from build123d import *

# Parameters (mm, degrees)
FILLET1_R = 1.5


with BuildPart() as part:
    # Sketch1 → Revolve1 (revolve)
    with BuildSketch(Plane.XY):
        with BuildLine():
            Line((29.062623268, -28.998781924), (35, -87.278860618))
            Line((35, -87.278860618), (50, -87.278860618))
            Line((50, -87.278860618), (50, -90.278860618))
            Line((50, -90.278860618), (70, -90.278860618))
            Line((70, -90.278860618), (70, -70.278860618))
            Line((70, -70.278860618), (50, -70.278860618))
            ThreePointArc((50, -70.278860618), (44.343145751, -67.935714867), (42, -62.278860618))
            Line((42, -62.278860618), (32, 52.5))
            Line((32, 52.5), (35, 52.5))
            Line((35, 52.5), (35, 92.5))
            Line((35, 92.5), (25, 92.5))
            Line((25, 92.5), (25, 17.342006044))
            Line((25, 17.342006044), (29.062623268, -28.998781924))
        make_face()
    revolve(axis=Axis((0, -90.278860618, 0), (0, 1, 0)))

    # Fillet1
    fillet1_edges = [part.edges().sort_by_distance(p)[0] for p in [
        (-50, -87.278860618, 0),
    ]]
    fillet(fillet1_edges, radius=FILLET1_R)


solid = part.part
Can you work these out from the model? Positions are in its coordinate system, mm. A direction names the side the tool comes from. Give positions to 0.01 mm unless a question says otherwise; leave off trailing zeros. Loops run counter-clockwise (first coordinate to the right, second up) from the corner with the lowest first, then second, coordinate; pieces in that order, holes last. Notation, with made-up numbers: (16, 7) -> (41, 7) arc R16 ccw to (41, 31) -> close; hole circle Ø1 at (35.25, 36). An arc over 180 degrees is marked (long way). Write item = value, one per line.
1) Suppose I cut it at A-A on z = 0. Write out the boundary of the cut face in (x, y).
Check result:
outline = (-70, -90.28) -> (-50, -90.28) -> (-50, -88.78) arc R1.5 cw to (-48.5, -87.28) -> (-35, -87.28) -> (-29.06, -29) -> (-25, 17.34) -> (-25, 92.5) -> (-35, 92.5) -> (-35, 52.5) -> (-32, 52.5) -> (-42, -62.28) arc R8 cw to (-50, -70.28) -> (-70, -70.28) -> close; (25, 17.34) -> (29.06, -29) -> (35, -87.28) -> (48.5, -87.28) arc R1.5 cw to (50, -88.78) -> (50, -90.28) -> (70, -90.28) -> (70, -70.28) -> (50, -70.28) arc R8 cw to (42, -62.28) -> (32, 52.5) -> (35, 52.5) -> (35, 92.5) -> (25, 92.5) -> close
2) Thinking about a two-plate mould opening in X: for faces 1 (the flat face through (-48, -70.279, -17)), 2 (the conical face through (19.85, -4.09, -31.14)), 3 (the cylindrical face through (47.69, -89.54, -15.02)), which applies, released by +X, released by -X, zero draft, split by the parting line, or undercut?
Check result:
face_1 = zero draft
face_2 = split by the parting line
face_3 = undercut
3) Suppose I cut it at B-B on x = 0. Write out the boundary of the cut face in (y, z).
Check result:
outline = (-90.28, -70) -> (-70.28, -70) -> (-70.28, -50) arc R8 cw to (-62.28, -42) -> (52.5, -32) -> (52.5, -35) -> (92.5, -35) -> (92.5, -25) -> (17.34, -25) -> (-29, -29.06) -> (-87.28, -35) -> (-87.28, -48.5) arc R1.5 cw to (-88.78, -50) -> (-90.28, -50) -> close; (-90.28, 50) -> (-88.78, 50) arc R1.5 cw to (-87.28, 48.5) -> (-87.28, 35) -> (-29, 29.06) -> (17.34, 25) -> (92.5, 25) -> (92.5, 35) -> (52.5, 35) -> (52.5, 32) -> (-62.28, 42) arc R8 cw to (-70.28, 50) -> (-70.28, 70) -> (-90.28, 70) -> close
4) For faces 4 (the cylindrical face through (-28, 73, 21)), 5 (the flat face through (-24, 92.5, -8)), 6 (the cylindrical face through (23.846, 54.395, -7.509)), 7 (the flat face through (-32, -87.279, -15)), 8 (the flat face through (-15.4, 52.5, 28.4)), which set-ups out of +Z, -Z, +X, -X, +Y, -Y let a thin tool reach every point of the face, with its end or its side?
Check result:
face_4 = +Y
face_5 = +Z, -Z, +X, -X, +Y
face_6 = +Y, -Y
face_7 = -Y
face_8 = none
5) Suppose I cut it at D-D on y = -20.5. Write out the boundary of the cut face in (x, z), then the cut area to 3 significant figures.
Check result:
outline = circle Ø76.72 at (0, 0); hole circle Ø56.64 at (0, 0)
area = 2,100 mm2
6) Suppose I cut it at C-C on y = 69.5. Write out the boundary of the cut face in (x, z).
Check result:
outline = circle Ø70 at (0, 0); hole circle Ø50 at (0, 0)
7) Will these pins go through, and if not, where does the flat tip stop? pin 1 (4 mm diameter, centred on x = -2, y = -11, fed in from +Z); pin 2 (10 mm diameter, centred on x = -10.5, z = -14.5, fed in from -Y); pin 3 (4 mm diameter, centred on y = -67.5, z = -6, fed in from +X); pin 4 (10 mm diameter, centred on x = 36, z = 44, fed in from +Y).
Check result:
pin_1 = 37.67
pin_2 = through
pin_3 = 46.18
pin_4 = -70.28
8) I need wall thicknesses on L1, parallel to Z at x = 0, y = 74; L2, parallel to X at y = -89, z = 0. Which ranges of each line are inside material? Lowest first, please. Write a range as from..to.
Check result:
L1 = -35..-25, 25..35
L2 = -70..-50, 50..70
